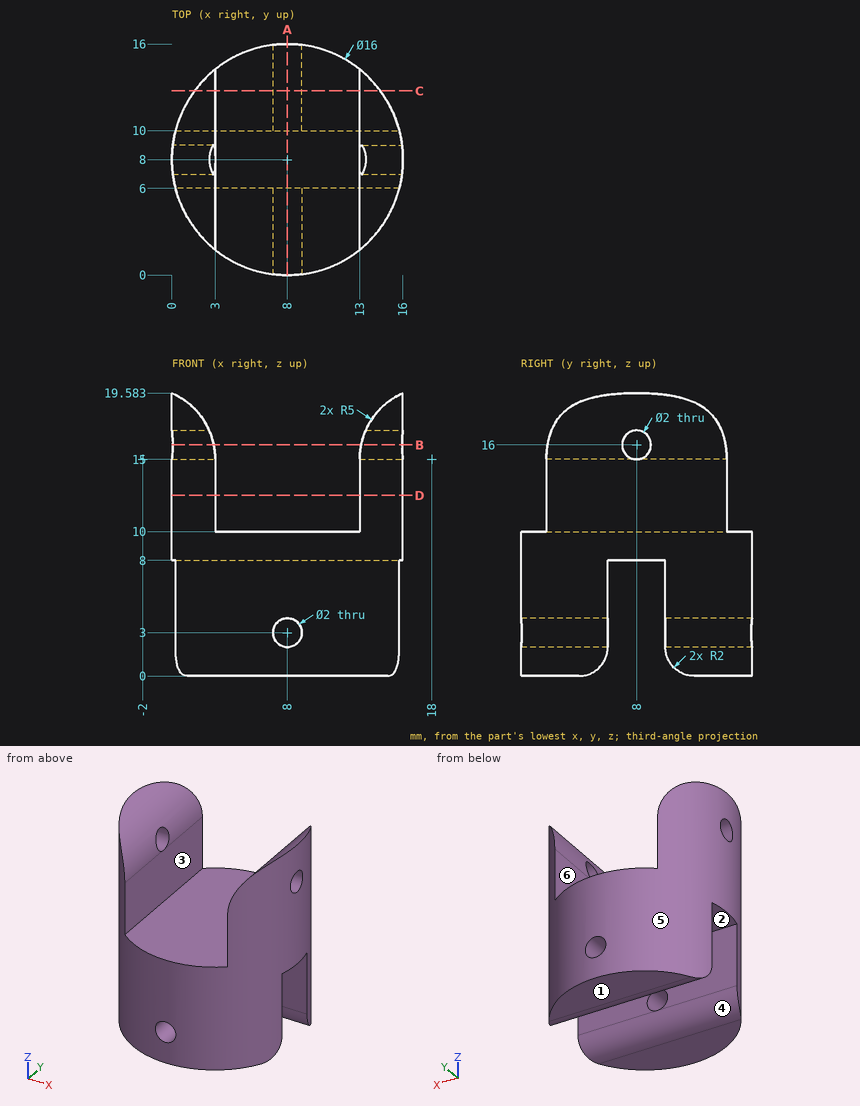
Source: three-view drawing plus pictorial views. Frame: mm from the lowest corner of the part. A direction names the side the tool comes from. Round coordinates to 2 decimals unless told otherwise and drop trailing zeros. Order: outer loops, then holes, each group sorted by start corner. A loop starts at its lowest first (then second) coordinate and runs counter-clockwise, first axis right, second up. Notation, with made-up numbers: M 52,5.25 L 76,5.25 A11 ccw 76,23.25 Z; hole C -5,-16 d10. An arc over 180 degrees is marked long. One line per item, written item: value.
(1) Pull-direction query (X, two-part tool) for the marked faces 4, 5 and 6; classes: pulls with the +X half, pulls with the -X half, needs draft (parallel to the pull), parting line crosses it, or undercut.
Result sheet:
face 4: needs draft
face 5: parting line crosses it
face 6: undercut
(2) Reachability of the marked faces 1, 2 and 3 from +Z, -Z, +X, -X, +Y, -Y: full face, straight path, thin tool, end or side. Return the list, or none.
Result sheet:
face 1: -Z, +X, -X, +Y, -Y
face 2: -Z, +X, -X
face 3: +Z, +Y, -Y
(3) Cut plane D-D (z = 12.5). Return the cut outline in (x, y) (1 decimal), and give its area (3 significant figures).
Result sheet:
outline: M 3,1.8 L 3,14.2 A8 ccw Z; M 13,1.8 A8 ccw 13,14.2 Z
area: 52.2 mm2
(4) Cut plane B-B (z = 16). Return the cut outline in (x, y).
Result sheet:
outline: M 0.06,7 A8 ccw 2.9,1.84 L 2.9,7 Z; M 0.06,9 L 2.9,9 L 2.9,14.16 A8 ccw Z; M 13.1,1.84 A8 ccw 15.94,7 L 13.1,7 Z; M 13.1,9 L 15.94,9 A8 ccw 13.1,14.16 Z
(5) Cut plane C-C (y = 12.75). Return the cut outline in (x, z).
Result sheet:
outline: M 1.56,0 L 14.44,0 L 14.44,18.51 A5 ccw 13,15.03 L 13,10 L 3,10 L 3,15.03 A5 ccw 1.56,18.51 Z; hole C 8,3 d2
(6) Cut plane A-A (x = 8). Give the number of separate pieces and of enclosed holes in the cut face, and give its area (3 significant figures).
Result sheet:
separate pieces: 3
enclosed holes: 0
area: 102 mm2
(7) Line query: probe 1 along Z at (x, y) = (8, 13.75); probe 2 along Z at (x, y) = (14.55, 8); probe 3 along X at (y, z) = (4, 17.25) (1 decimal). Output: solid intervals per line, ascending. Write a range as [from, to].
Result sheet:
probe 1: [0, 2], [4, 10]
probe 2: [8, 15], [17, 18.62]
probe 3: [1.1, 2.5], [13.5, 14.9]
(8) Pin query (flat end, axial travel): P1, Ø1, axis at x = 4, y = 2, coming from the +Z side; P2, Ø3, axis at x = 4, z = 5, coming from the +Y side; P3, Ø2, axis at x = 6, z = 4, coming from the -Y side. Return the tip coordinate at first contact, or that it passes through.
Result sheet:
P1: z = 10
P2: y = 15.6
P3: y = 0.06
